Input: part model. Units: mm. Frame: model coordinates. Face numbers are marked on the shaded views. A direction names the side the tool comes from. Coordinates: 2 decimals unless noted, no trailing zeros. Write each loop counter-clockwise with the first axis right and the second up, starting at its lowest first coordinate (ties: lowest second). Pieces come first, ordered by that corner, then holes.
1) Section query C-C (y = 13). Output: boundary loops of the cut face in (x, z).
2) Section query B-B (x = 0). Output: boundary loops of the cut face in (y, z), then the cut area to 3 significant figures.
3) Line query: L1, parallel to Y at x = 4, z = 7; L2, parallel to X at y = 37.5, z = 6.5; L3, parallel to Z at x = 3, y = 8. Output: solid intervals per line, ascending.
4) Draft query along Z for the marked faces 5, 6, 7 and 8. Return one class per face: pulls with the +Z half, pulls with the -Z half, needs draft (parallel to the pull), parting line crosses it, or undercut.
5) Set-up query: the marked faces 1, 2, 3 and 4. Return all of +Z, -Z, +X, -X, +Y, -Y with unobstructed straight access to the full face (end or side cutting, diameter ignored); none if empty.
6) Section query A-A (y = 34). Output: boundary loops of the cut face in (x, z).
7) Pin query (flat end, axial travel): pin 1 Ø1.5 at (x, y) = (7.5, 14.5) entering from -Z; pin 2 Ø1 at (y, z) = (2.5, 14.5) entering from +X; pin 3 Ø6 at (y, z) = (22, -0.5) entering from -X. Return the tip coordinate at first contact, or that it passes through.
8) Section query D-D (y = 26). Output: boundary loops of the cut face in (x, z), then the cut area to 3 significant figures.
from build123d import *

# Parameters (mm, degrees)
SKETCH_1_R           = 16
EXTRUDE_1_DEPTH      = 48
EXTRUDE_1_TAPER      = 5
SKETCH_2_R           = 9
CUT_EXTRUDE_1_DEPTH  = 3
CUT_EXTRUDE_1_DRAFT  = 6
CUT_EXTRUDE_2_DEPTH  = 2
SKETCH_6_R           = 12.5
CUT_EXTRUDE_3_DEPTH  = 43
CUT_EXTRUDE_3_TAPER  = 5
EXTRUDE_2_DEPTH      = 3
EXTRUDE_3_DEPTH      = 4
EXTRUDE_3_DEPTH_BACK = 1
CUT_EXTRUDE_5_DEPTH  = 5


with BuildPart() as part:
    # 草图1 → 凸台-拉伸1 (new body)
    with BuildSketch(Plane(origin=(0, 0, 0), x_dir=(1, 0, 0), z_dir=(0, 1, 0))):
        Circle(SKETCH_1_R)
    extrude(amount=EXTRUDE_1_DEPTH, taper=EXTRUDE_1_TAPER)


with BuildPart() as cut_extrude_1_tool:
    # 草图2 → 切除-拉伸1 (with draft: the straight prism first)
    with BuildSketch(Plane(origin=(0, 48, 0), x_dir=(1, 0, 0), z_dir=(0, 1, 0))):
        Circle(SKETCH_2_R)
    extrude(amount=-CUT_EXTRUDE_1_DEPTH)
    # 切除-拉伸1: the draft: its side faces are tilted about the plane it starts from
    cut_extrude_1_sides = [cut_extrude_1_tool.faces().sort_by_distance(p)[0] for p in [
        (-9, 46.5, 0),
    ]]
    draft(cut_extrude_1_sides, Plane(origin=(0, 48, 0), x_dir=(1, 0, 0), z_dir=(0, 1, 0)), CUT_EXTRUDE_1_DRAFT)


with BuildPart() as part_1:
    add(part.part)

    # 切除-拉伸1: cut by cut_extrude_1_tool
    add(cut_extrude_1_tool.part, mode=Mode.SUBTRACT)

    # 草图3 → 切除-拉伸2 (cut)
    with BuildSketch(Plane.XY.offset(16)):
        with BuildLine():
            Line((-4.721374977, 0), (4.721374977, 0))
            Line((4.721374977, 0), (4.721374977, 9.932117857))
            ThreePointArc((4.721374977, 9.932117857), (0, 14.653492833), (-4.721374977, 9.932117857))
            Line((-4.721374977, 9.932117857), (-4.721374977, 0))
        make_face()
    extrude(amount=-CUT_EXTRUDE_2_DEPTH, mode=Mode.SUBTRACT)

    # 草图6 → 切除-拉伸3 (cut)
    with BuildSketch(Plane(origin=(0, 0, 0), x_dir=(1, 0, 0), z_dir=(0, 1, 0))):
        Circle(SKETCH_6_R)
    extrude(amount=CUT_EXTRUDE_3_DEPTH, taper=CUT_EXTRUDE_3_TAPER, mode=Mode.SUBTRACT)

    # 草图8 → 凸台-拉伸2 (add)
    with BuildSketch(Plane(origin=(0, 40, 0), x_dir=(1, 0, 0), z_dir=(0, 1, 0))):
        with BuildLine():
            Line((-11.961452846, -10.626553807), (-9.345224038, -8.302296331))
            ThreePointArc((-9.345224038, -8.302296331), (0, -12.500453459), (9.345224038, -8.302296331))
            Line((9.345224038, -8.302296331), (11.961452846, -10.626553807))
            ThreePointArc((11.961452846, -10.626553807), (0, -16), (-11.961452846, -10.626553807))
        make_face()
    extrude(amount=-EXTRUDE_2_DEPTH)

    # 草图9 → 凸台-拉伸3 (add, two sides: drawn at the far end of the back side and taken through both)
    with BuildSketch(Plane(origin=(15.878462024, 1.389185421, 0), x_dir=(0, 0, -1), z_dir=(0.9961946980917457, 0.0871557427476584, 0)).offset(-EXTRUDE_3_DEPTH_BACK)):
        Polygon((-2.592399587, 34.872205125), (2.592399587, 34.872205125), (3.662079691, 16.297695401), (-3.662079691, 16.297695401), align=None)
    extrude(amount=EXTRUDE_3_DEPTH + EXTRUDE_3_DEPTH_BACK)

    # 草图11 → 切除-拉伸5 (cut)
    with BuildSketch(Plane(origin=(20.768531886, 3.289412299, 0), x_dir=(0, 0, -1), z_dir=(0.9876883405951382, 0.15643446504022776, 0))):
        Polygon((2.592399587, 33.486979454), (-2.592399587, 33.486979454), (-3.662079691, 14.86711267), (3.662079691, 14.86711267), align=None)
    extrude(amount=CUT_EXTRUDE_5_DEPTH, mode=Mode.SUBTRACT)

    # 镜向1: part across plane


with BuildPart() as part_2:
    add(part_1.part)
    add(part_1.part.mirror(Plane(origin=(0, 0, 0), x_dir=(0, 0, 1), z_dir=(1, 0, 0))))


solid = part_2.part
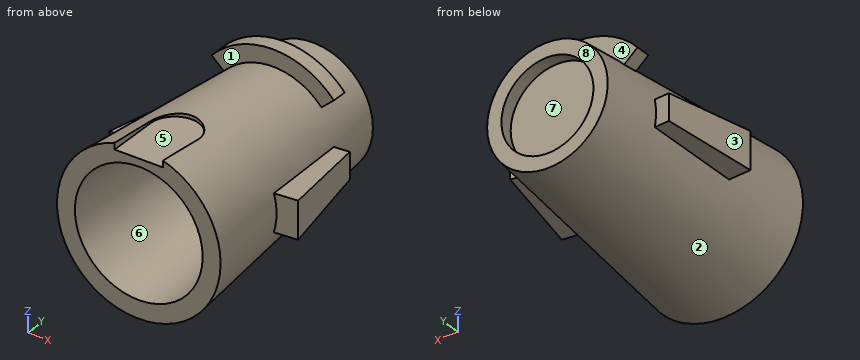
Answer:
1. outline: (-3.59, 14) - (-3.59, 14.42) arc R14.86 ccw (long way) to (3.59, 14.42) - (3.59, 14) - close; hole circle Ø22.73 at (0, 0)
2. outline: (0, -16) - (48, -11.8) - (48, -9) - (45, -9.32) - (45, 9.32) - (48, 9) - (48, 11.8) - (40, 12.5) - (40, 16) - (37, 16) - (37, 12.76) - (14.65, 14.72) - (14.65, 14) - (0, 14) - (0, 12.5) - (43, 8.74) - (43, -8.74) - (0, -12.5) - close
2. area: 356 mm2
3. L1: y = 43 to 45
3. L2: x = -10.93 to -6.54, 6.54 to 10.93
3. L3: z = -15 to -11.41, 11.41 to 14
4. face 5: pulls with the +Z half
4. face 6: undercut
4. face 7: undercut
4. face 8: needs draft
5. face 1: +Z
5. face 2: none
5. face 3: +Z, -Z, -X, +Y
5. face 4: +Z, +Y
6. outline: (-15.9, -2.73) - (-12.74, -2.71) arc R13.03 ccw to (12.74, -2.71) - (15.9, -2.73) - (15.9, 2.73) - (12.74, 2.71) arc R13.03 ccw to (-12.74, 2.71) - (-15.9, 2.73) - close; hole circle Ø19.05 at (0, 0)
7. pin 1: stops at z = -13.1
7. pin 2: stops at x = 7.29
7. pin 3: stops at x = -18.28
8. outline: (-17.17, -3.2) - (-13.35, -3.18) arc R13.73 ccw to (13.35, -3.18) - (17.17, -3.2) - (17.17, 3.2) - (13.35, 3.18) arc R13.73 ccw to (-13.35, 3.18) - (-17.17, 3.2) - close; hole circle Ø20.45 at (0, 0)
8. area: 309 mm2
